from build123d import *

# Parameters (mm, degrees)
SWEEP3_PROFILE_R    = 4
SWEEP4_PROFILE_R    = 5.5
SKETCH45_R          = 2.25
CUT_EXTRUDE2_DEPTH  = 337.377466094
SWEEP5_PROFILE_R    = 0.25
SWEEP6_PROFILE_R    = 0.25
SKETCH72_W          = 4.5
SKETCH72_H          = 20
CUT_EXTRUDE6_DEPTH  = 20
SKETCH77_R          = 1
BOSS_EXTRUDE1_DEPTH = 1


with BuildPart() as part:
    # Sweep3: sweep along a path in Sketch31
    with BuildLine(Plane.XY) as sweep3_path:
        Line((0, 0), (0, 35.470165431))
    # Sweep3 profile (on start of the path) → Sweep3 (sweep)
    with BuildSketch(Plane.ZX):
        Circle(SWEEP3_PROFILE_R)
    sweep(path=sweep3_path.line)

    # Sweep4: sweep along a path in Sketch38
    with BuildLine(Plane.XY) as sweep4_path:
        Line((0, 35.470165431), (0, 336.287525335))
    # Sweep4 profile (on start of the path) → Sweep4 (sweep)
    with BuildSketch(Plane.ZX.offset(35.470165431)):
        Circle(SWEEP4_PROFILE_R)
    sweep(path=sweep4_path.line)

    # Sketch45 → Cut-Extrude2 (cut, through all)
    with BuildSketch(Plane(origin=(0, 0, 0), x_dir=(1, 0, 0), z_dir=(0, 1, 0))):
        with Locations(Location((0, 0, 0), (0, 0, 270))):
            Circle(SKETCH45_R)
    extrude(amount=CUT_EXTRUDE2_DEPTH, mode=Mode.SUBTRACT)

    # Sweep5: sweep along a curve in space
    with BuildLine() as sweep5_path:
        Line((4.125, 336.287525335, 5.531e-06), (4.125, 337.787525335, 5.531e-06))
    # Sweep5 profile (on start of the path) → Sweep5 (sweep)
    with BuildSketch(Plane(origin=(4.125, 336.287525335, 5.531e-06), x_dir=(0, 0, 1), z_dir=(0, 1, 0))):
        Circle(SWEEP5_PROFILE_R)
    sweep(path=sweep5_path.line)

    # Sweep6: sweep along a curve in space
    with BuildLine() as sweep6_path:
        Line((-4.125, 336.287525335, 9.31e-07), (-4.125, 337.787525335, 9.31e-07))
    # Sweep6 profile (on start of the path) → Sweep6 (sweep)
    with BuildSketch(Plane(origin=(-4.125, 336.287525335, 9.31e-07), x_dir=(0, 0, 1), z_dir=(0, 1, 0))):
        Circle(SWEEP6_PROFILE_R)
    sweep(path=sweep6_path.line)

    # Sketch72 → Cut-Extrude6 (cut)
    with BuildSketch(Plane(origin=(0, 0, 0), x_dir=(0, 0, -1), z_dir=(1, 0, 0))):
        with Locations((-0.068000409, 19.236124066)):
            Rectangle(SKETCH72_W, SKETCH72_H)
    extrude(amount=CUT_EXTRUDE6_DEPTH, mode=Mode.SUBTRACT)

    # Sketch77 → Boss-Extrude1 (add)
    with BuildSketch(Plane(origin=(0, 336.287525335, 0), x_dir=(1, 0, 0), z_dir=(0, 1, 0))):
        with Locations(Location((-4, -9.03e-07, 0), (0, 0, 270))):
            Circle(SKETCH77_R)
        with Locations(Location((4, -5.363e-06, 0), (0, 0, 270))):
            Circle(SKETCH77_R)
    extrude(amount=BOSS_EXTRUDE1_DEPTH)


solid = part.part
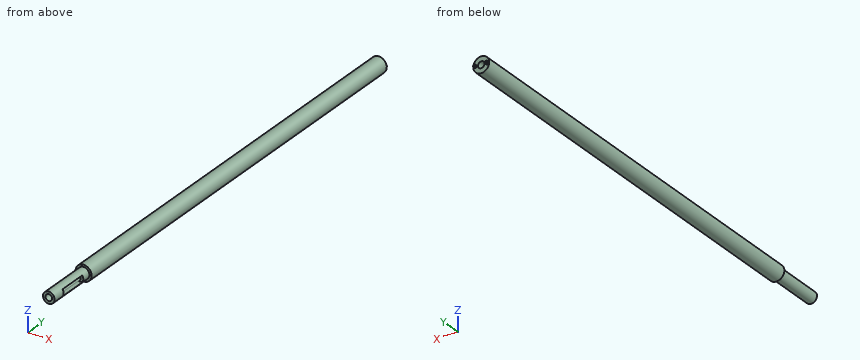
CAD build for the part. Positions are in the model's coordinates, mm. Round coordinates to 2 decimals unless told otherwise and drop trailing zeros. Write each loop counter-clockwise with the first axis right and the second up, starting at its lowest first coordinate (ties: lowest second). Pieces come first, ordered by that corner, then holes.
(1) Slice it at A-A, the plane y = 210. Write the cut outline in (x, z).
(2) Probe line 1 along X through (y, z) = (161, 0); line 2 along Y through (x, z) = (2.25, -2); line 3 along Y through (x, z) = (-1.5, -1.75). List the from-to ranges inside material, lowest first.
(3) Drop flat-ended pins along their axis: P1, Ø0.8, axis at x = 2, y = 22.5, coming from the +Z side; P2, Ø4, axis at x = 4.5, y = 98.5, coming from the +Z side; P3, Ø2, axis at y = 251.5, z = -3.5, coming from the +X side. Give the stop position or say it passes through.
From the geometry:
1. outline: circle Ø11 at (0, 0); hole circle Ø4.5 at (0, 0)
2. line 1: x = -5.5 to -2.25, 2.25 to 5.5
2. line 2: y = 0 to 9.24, 29.24 to 336.29
2. line 3: y = 0 to 336.29
3. P1: stops at z = 3.67
3. P2: stops at z = 4.9
3. P3: stops at x = 4.9
